Autodesk Inventor part; units mm, degrees
ref_plane "YZ Plane" through (0, 0, 0) normal (1, 0, 0) x (0, 1, 0)
ref_plane "XZ Plane" through (0, 0, 0) normal (0, 1, 0) x (-1, 0, 0)
ref_plane "XY Plane" through (0, 0, 0) normal (0, 0, 1) x (1, 0, 0)
sketch "Sketch1" plane through (0, 0, 0) normal (0, 0, 1) x (1, 0, 0)
  line L0 (0, 0) -> (88.9, 0)
  line L1 (88.9, 0) -> (88.9, -25.4)
  line L2 (88.9, -25.4) -> (0, -25.4)
  line L3 (0, -25.4) -> (0, 0)
  dimension "d0" = 88.9
  dimension "d1" = 25.4
extrude "Extrusion1" add sketch "Sketch1" against normal blind 114.3
sketch "Sketch2" plane through (0, 0, 0) normal (0, 1, 0) x (1, 0, 0)
  line L0 (0, 0) -> (88.9, 0)
  line L1 (88.9, 0) -> (88.9, 114.3)
  line L2 (0, 114.3) -> (88.9, 114.3)
  line L3 (0, 0) -> (0, 114.3)
  line L4 (3.175, 3.175) -> (85.725, 3.175)
  line L5 (85.725, 3.175) -> (85.725, 111.125)
  line L6 (85.725, 111.125) -> (3.175, 111.125)
  line L7 (3.175, 111.125) -> (3.175, 3.175)
  dimension "d4" = 3.175
  dimension "d5" = 3.175
  dimension "d6" = 3.175
  dimension "d7" = 3.175
extrude "Extrusion2" cut sketch "Sketch2" against normal blind 22.225 contours L7 L6 L5 L4
sketch "Sketch3" plane through (0, 0, 0) normal (0, 0, 1) x (1, 0, 0)
  line L0 (0, -25.4) -> (0, 0)
  line L1 (88.9, 0) -> (88.9, -25.4)
  line L2 (0, -25.4) -> (0, 0)
  line L3 (88.9, 0) -> (88.9, -25.4)
  line L4 (1.5875, -2.3041) -> (87.3125, -2.3041)
  line L5 (87.3125, -2.3041) -> (87.3125, -5.4791)
  line L6 (87.3125, -5.4791) -> (1.5875, -5.4791)
  line L7 (1.5875, -5.4791) -> (1.5875, -2.3041)
  dimension "d46" = 3.175
  dimension "d47" = 1.5875
  dimension "d49" = 1.5875
extrude "Extrusion3" cut sketch "Sketch3" against normal blind 112.7125
sketch "Sketch5" plane through (0, 0, 0) normal (0, 1, 0) x (1, 0, 0)
  line L0 (3.175, 3.175) -> (3.175, 111.125)
  line L1 (3.175, 3.175) -> (12.7, 3.175)
  line L2 (12.7, 3.175) -> (12.7, 12.7)
  line L3 (12.7, 12.7) -> (3.175, 12.7)
  line L4 (3.175, 12.7) -> (3.175, 3.175)
  line L5 (85.725, 3.175) -> (76.2, 3.175)
  line L6 (76.2, 3.175) -> (76.2, 12.7)
  line L7 (76.2, 12.7) -> (85.725, 12.7)
  line L8 (85.725, 12.7) -> (85.725, 3.175)
  dimension "d64" = 9.525
  dimension "d67" = 9.525
  dimension "d68" = 9.525
  dimension "d69" = 9.525
extrude "Extrusion4" add sketch "Sketch5" against normal blind 6.35
sketch "Sketch6" plane through (0, 0, 0) normal (0, 0, 1) x (1, 0, 0)
  line L0 (12.7, -6.7991) -> (3.175, -6.7991)
  line L1 (3.175, -6.7991) -> (3.175, -16.3241)
  line L2 (3.175, -16.3241) -> (12.7, -16.3241)
  line L3 (12.7, -16.3241) -> (12.7, -6.7991)
  line L4 (76.2, -6.7991) -> (85.725, -6.7991)
  line L5 (85.725, -6.7991) -> (85.725, -16.3241)
  line L6 (85.725, -16.3241) -> (76.2, -16.3241)
  line L7 (76.2, -16.3241) -> (76.2, -6.7991)
  line L8 (87.3125, -5.4791) -> (1.5875, -5.4791)
  line L9 (0, -25.4) -> (0, 0)
  line L10 (88.9, 0) -> (88.9, -25.4)
  dimension "d70" = 9.525
  dimension "d71" = 9.525
  dimension "d72" = 9.525
  dimension "d73" = 9.525
  dimension "d76" = 1.32
  dimension "d77" = 1.32
  dimension "d78" = 3.175
  dimension "d79" = 3.175
extrude "Extrusion5" add sketch "Sketch6" along normal blind 1.5875
equation "\"d49\" = d47"
equation "\"d65\" = d62"
equation "\"d73\" = d71"
equation "\"d79\" = d78"
properties part number "Electronics Container"
The model under review builds one solid part; all positions refer to its coordinate system, in mm. A direction names the side the tool comes from. Round coordinates to 2 decimals unless told otherwise and drop trailing zeros. Loops run counter-clockwise (first coordinate to the right, second up) from the corner with the lowest first, then second, coordinate; pieces in that order, holes last. Notation, with made-up numbers: (55, 60.25) -> (92, 60.25) arc R26 ccw to (92, 99.25) -> close; hole circle Ø1 at (9, 73). An arc over 180 degrees is marked (long way). Answer as a JSON object with one key per item and string values. Group by question number.
1) Mouldability with a two-part tool opening along Z and no side actions: class faces 1 (the face through (3.175, -14, -58)), 2 (the face through (87.312, -4, -56)), 3 (the face through (44, -22.225, -58)), 4 (the face through (44, -13, -114.3)) as released by +Z, released by -Z, zero draft, split by the parting line, or undercut.
2) For faces 5 (the face through (45, -25.4, -56)), 6 (the face through (1.588, -4, -56)), 7 (the face through (81, -3, -12.7)), 8 (the face through (81, -6.35, -8)), list the 3-axis set-ups (+Z, -Z, +X, -X, +Y, -Y) from which the entire face can be reached by the end or side of a thin tool; tool diameter is ignored.
3) For line 1 (X direction, y = -7, z = -38.5) (3 decimals); line 2 (Z direction, x = 23.5, y = -10.25) (3 decimals); line 3 (Y direction, x = 6, z = -8) (3 decimals), list the stretches that pass through material, from the lowest coordinate up. Write a range as [from, to].
4) We need section D-D on z = -89. Write out the cut boundary in (x, y) (1 decimal).
5) We need section C-C on z = -10. Give the number of separate pieces and of enclosed holes in the cut face, then the cut area to 3 significant figures.
6) We need section A-A on x = 61.5. Write out the cut boundary in (y, z) (1 decimal), then the cut area to 3 significant figures.
7) For pin 1 Ø1 at (x, y) = (81.5, -4.5) entering from +Z (3 decimals); pin 2 Ø0.5 at (y, z) = (-13.5, 1) entering from +X (3 decimals); pin 3 Ø2 at (x, z) = (27.5, -75) entering from +Y (3 decimals), all flat-tipped, find the tip position at first contact; note any pin that passes through.
8) We need section B-B on y = -18. Write out the cut boundary in (x, z) (3 decimals), then the cut area to 3 significant figures.
Result set:
{
 "1": {"face 1": "undercut", "face 2": "zero draft", "face 3": "undercut", "face 4": "released by -Z"},
 "2": {"face 5": "+Z, -Z, +X, -X, -Y", "face 6": "+Z", "face 7": "+Y", "face 8": "none"},
 "3": {"line 1": "[0, 3.175], [85.725, 88.9]", "line 2": "[-114.3, -111.125], [-3.175, 0]", "line 3": "[-25.4, -22.225], [-6.35, 0]"},
 "4": {"outline": "(0, -25.4) -> (88.9, -25.4) -> (88.9, 0) -> (85.7, 0) -> (85.7, -2.3) -> (87.3, -2.3) -> (87.3, -5.5) -> (85.7, -5.5) -> (85.7, -22.2) -> (3.2, -22.2) -> (3.2, -5.5) -> (1.6, -5.5) -> (1.6, -2.3) -> (3.2, -2.3) -> (3.2, 0) -> (0, 0) -> close"},
 "5": {"separate pieces": "1", "enclosed holes": "2", "area": "534 mm²"},
 "6": {"outline": "(-25.4, -114.3) -> (0, -114.3) -> (0, -111.1) -> (-2.3, -111.1) -> (-2.3, -112.7) -> (-5.5, -112.7) -> (-5.5, -111.1) -> (-22.2, -111.1) -> (-22.2, -3.2) -> (-5.5, -3.2) -> (-5.5, 0) -> (-25.4, 0) -> close; (-2.3, -3.2) -> (0, -3.2) -> (0, 0) -> (-2.3, 0) -> close", "area": "489 mm²"},
 "7": {"pin 1": "z = -3.175", "pin 2": "x = 85.725", "pin 3": "y = -22.225"},
 "8": {"outline": "(0, -114.3) -> (88.9, -114.3) -> (88.9, 0) -> (0, 0) -> close; hole (3.175, -111.125) -> (85.725, -111.125) -> (85.725, -3.175) -> (3.175, -3.175) -> close", "area": "1,250 mm²"}
}
